Build history of the part. All positions in model axes, mm. Face numbers are marked on the shaded views. A direction names the side the tool comes from. Give positions to 0.01 mm unless a question says otherwise; leave off trailing zeros. Loops run counter-clockwise (first coordinate to the right, second up) from the corner with the lowest first, then second, coordinate; pieces in that order, holes last. Notation, with made-up numbers: M -13,6 L 31,6 A11 cw 31,27 Z; hole C 49.25,81.5 d9. An arc over 180 degrees is marked long. Put each result on its own line as item: value.
```python
from build123d import *

# Parameters (mm, degrees)
F0_R      = 44.45
F1_DEPTH  = 88.9
F2_R      = 6.35
F3_DEPTH  = 25.4
F5_DEPTH  = 25.4
F6_R      = 6.35
F7_DEPTH  = 25.4
F10_DEPTH = 22.225
F12_R     = 44.45
F12_R_2   = 41.91
F13_DEPTH = 0.127
F15_R     = 48.4692120424
F15_R_2   = 41.275
F16_DEPTH = 25.4


with BuildPart() as f1:
    # F0 (on Front) → F1 (new body)
    with BuildSketch(Plane.XZ):
        Circle(F0_R)
    extrude(amount=F1_DEPTH)

    # F2 (on face) → F3 (cut)
    with BuildSketch(Plane.XZ.offset(88.9)):
        Circle(F2_R)
    extrude(amount=-F3_DEPTH, mode=Mode.SUBTRACT)

    # F4 (on face) → F5 (cut)
    with BuildSketch(Plane.XZ.offset(88.9)):
        with BuildLine():
            ThreePointArc((19.05, 40.1609262841), (0, 44.45), (-19.05, 40.1609262841))
            Line((-19.05, 40.1609262841), (19.05, 40.1609262841))
        make_face()
    extrude(amount=-F5_DEPTH, mode=Mode.SUBTRACT)

    # F6 (on face) → F7 (cut)
    with BuildSketch(Plane.XY.offset(40.1609262841)):
        with Locations((0, -76.2)):
            Circle(F6_R)
    extrude(amount=-F7_DEPTH, mode=Mode.SUBTRACT)

    # F9 (on offset) → F10 (cut)
    with BuildSketch(Plane.XZ.offset(85.725)):
        with BuildLine():
            Line((18.1031520743, 36.9859262841), (-18.1031520743, 36.9859262841))
            ThreePointArc((-18.1031520743, 36.9859262841), (0, -41.1786699411), (18.1031520743, 36.9859262841))
        make_face()
    extrude(amount=-F10_DEPTH, mode=Mode.SUBTRACT)

    # F12 (on offset) → F13 (cut)
    with BuildSketch(Plane.XZ.offset(60.325)):
        Circle(F12_R)
        Circle(F12_R_2, mode=Mode.SUBTRACT)
    extrude(amount=-F13_DEPTH, mode=Mode.SUBTRACT)

    # F15 (on offset) → F16 (cut)
    with BuildSketch(Plane.XZ.offset(6.35)):
        Circle(F15_R)
        Circle(F15_R_2, mode=Mode.SUBTRACT)
    extrude(amount=F16_DEPTH, mode=Mode.SUBTRACT)


solid = f1.part
```
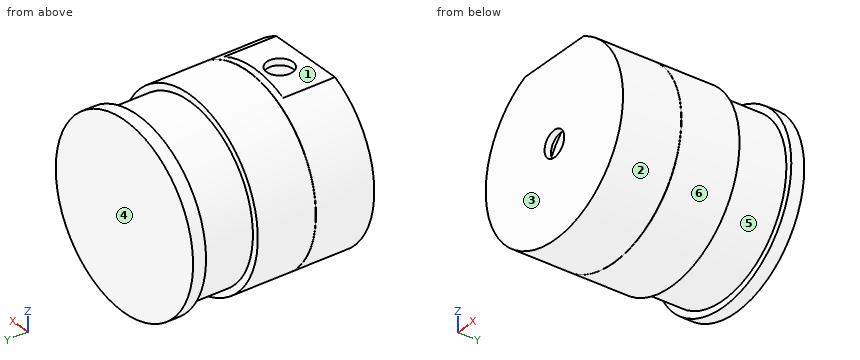
Q1. Slice it at B-B (z = 0). List the corners of the cut face in (x, y) (3 decimals).
Here are the results:
outline: M -44.45,-88.9 L -6.35,-88.9 L -6.35,-85.725 L -41.179,-85.725 L -41.179,-63.5 L 41.179,-63.5 L 41.179,-85.725 L 6.35,-85.725 L 6.35,-88.9 L 44.45,-88.9 L 44.45,-60.325 L 41.91,-60.325 L 41.91,-60.198 L 44.45,-60.198 L 44.45,-31.75 L 41.275,-31.75 L 41.275,-6.35 L 44.45,-6.35 L 44.45,0 L -44.45,0 L -44.45,-6.35 L -41.275,-6.35 L -41.275,-31.75 L -44.45,-31.75 L -44.45,-60.198 L -41.91,-60.198 L -41.91,-60.325 L -44.45,-60.325 Z
Q2. Probe line 1 (Z direction, x = 0, y = -88.2); line 2 (Y direction, x = -35, z = -5.5) (3 decimals); line 3 (X direction, y = -77, z = 0). List the from-to ranges inside material, lowest first. Write a range as from..to.
Here are the results:
line 1: -44.45..-6.35, 6.35..40.16
line 2: -88.9..-85.725, -63.5..0
line 3: -44.45..-41.18, 41.18..44.45
Q3. Tool access for the marked faces 1 and 2: list every direction of +Z, -Z, +X, -X, +Y, -Y with a clear straight run to the whole face (end or side of a thin tool).
Here are the results:
face 1: +Z, +X, -X, -Y
face 2: +Y, -Y
Q4. Mould opens along Y. For the marked faces 3, 4, 5 and 6 say: pulls with the +Y half, pulls with the -Y half, needs draft (parallel to the pull), parting line crosses it, or undercut.
Here are the results:
face 3: pulls with the -Y half
face 4: pulls with the +Y half
face 5: undercut
face 6: needs draft
Q5. Slice it at C-C (x = -27.5). List the corners of the cut face in (y, z) (3 decimals), and give its area (3 significant figures).
Here are the results:
outline: M -88.9,-34.922 L -60.325,-34.922 L -60.325,-31.626 L -60.198,-31.626 L -60.198,-34.922 L -31.75,-34.922 L -31.75,-30.779 L -6.35,-30.779 L -6.35,-34.922 L 0,-34.922 L 0,34.922 L -6.35,34.922 L -6.35,30.779 L -31.75,30.779 L -31.75,34.922 L -60.198,34.922 L -60.198,31.626 L -60.325,31.626 L -60.325,34.922 L -88.9,34.922 Z; hole M -85.725,-30.65 L -63.5,-30.65 L -63.5,30.65 L -85.725,30.65 Z
area: 4,640 mm²
Q6. Drop flat-ended pins along their axis: pin 1 Ø1.3 at (x, z) = (6, 43) entering from -Y; pin 2 Ø20.5 at (x, y) = (8.5, -75) entering from +Z; pin 3 Ø4 at (y, z) = (-13.5, 33) entering from +X. Give the stop position or say it passes through.
Here are the results:
pin 1: y = -63.5
pin 2: z = 40.16
pin 3: x = 27.25
Q7. Slice it at D-D (y = -76.2). List the corners of the cut face in (x, z), and give its area (3 significant figures).
Here are the results:
outline: M -19.05,40.16 A44.45 ccw long 19.05,40.16 L 6.35,40.16 L 6.35,36.99 L 18.1,36.99 A41.18 cw long -18.1,36.99 L -6.35,36.99 L -6.35,40.16 Z
area: 832 mm²
